Part model, mm, in its own coordinate system. Face numbers are marked on the shaded views. Round coordinates to 2 decimals unless told otherwise and drop trailing zeros. Loops run counter-clockwise (first coordinate to the right, second up) from the corner with the lowest first, then second, coordinate; pieces in that order, holes last. Notation, with made-up numbers: M 80,34.5 L 135,34.5 A20 ccw 135,39.5 Z; hole C 78,-17.5 d7. An arc over 180 degrees is marked long. Put each result on its own line as item: value. Start each with the question number.
1) Slice it at A-A on y = -4.5. Give the cut face in (x, z) (3 decimals).
2) Probe line 1 along Y through (x, z) = (0, 4.25) (3 decimals); line 2 along X through (y, z) = (-6, 4); line 3 along X through (y, z) = (6.5, 5.5). List the from-to ranges inside material, lowest first.
3) Slice it at D-D on y = 7.6. Give the cut face in (x, z) (3 decimals).
4) Drop flat-ended pins along their axis: pin 1 Ø8 at (x, y) = (2.5, -9) entering from -Z; pin 2 Ø2.5 at (x, y) = (0, -4.5) entering from +Z. Give the stop position or say it passes through.
5) Slice it at B-B on x = 0. Give the cut face in (y, z) (3 decimals), then the cut area to 3 significant figures.
6) Pull direction X, two halves, no side cores. Call the marked faces 1, 2 and 3: +X half, -X half, draft (parallel to the pull), parting line (faces both ways), or undercut.
7) Slice it at C-C on z = 1. Give the cut face in (x, y) (3 decimals), then the cut area to 3 significant figures.
```python
from build123d import *

# Parameters (mm, degrees)
F0_W     = 20
F0_H     = 25
F0_R     = 2.125
F1_DEPTH = 6.2
F2_R     = 8


with BuildPart() as f1:
    # F0 (on Top) → F1 (new body)
    with BuildSketch(Plane.XY):
        Rectangle(F0_W, F0_H)
        with Locations((0, -4.5)):
            Circle(F0_R, mode=Mode.SUBTRACT)
        with Locations((0, 7.6)):
            Circle(F0_R, mode=Mode.SUBTRACT)
    extrude(amount=F1_DEPTH)

    # F2
    f2_edges = [f1.edges().sort_by_distance(p)[0] for p in [
        (-10, 12.5, 3.1),
        (10, 12.5, 3.1),
    ]]
    fillet(f2_edges, radius=F2_R)


solid = f1.part
```
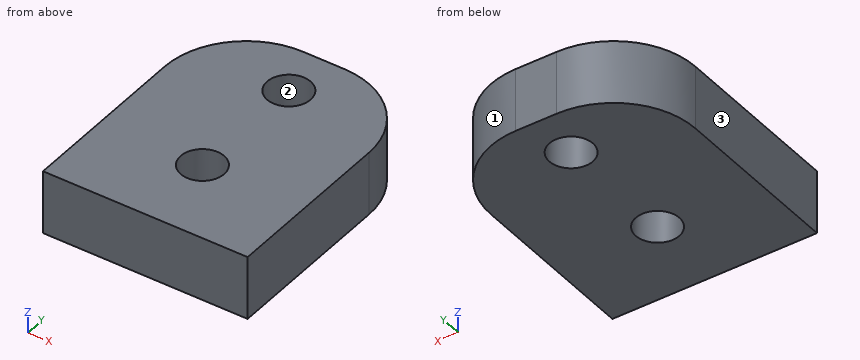
Recorded:
1. outline: M -10,0 L -2.125,0 L -2.125,6.2 L -10,6.2 Z; M 2.125,0 L 10,0 L 10,6.2 L 2.125,6.2 Z
2. line 1: y = -12.5 to -6.625, -2.375 to 5.475, 9.725 to 12.5
2. line 2: x = -10 to -1.51, 1.51 to 10
2. line 3: x = -9.75 to -1.82, 1.82 to 9.75
3. outline: M -9.375,0 L -2.125,0 L -2.125,6.2 L -9.375,6.2 Z; M 2.125,0 L 9.375,0 L 9.375,6.2 L 2.125,6.2 Z
4. pin 1: stops at z = 0
4. pin 2: passes through
5. outline: M -12.5,0 L -6.625,0 L -6.625,6.2 L -12.5,6.2 Z; M -2.375,0 L 5.475,0 L 5.475,6.2 L -2.375,6.2 Z; M 9.725,0 L 12.5,0 L 12.5,6.2 L 9.725,6.2 Z
5. area: 102 mm2
6. face 1: +X half
6. face 2: undercut
6. face 3: -X half
7. outline: M -10,-12.5 L 10,-12.5 L 10,4.5 A8 ccw 2,12.5 L -2,12.5 A8 ccw -10,4.5 Z; hole C 0,-4.5 d4.25; hole C 0,7.6 d4.25
7. area: 444 mm2
